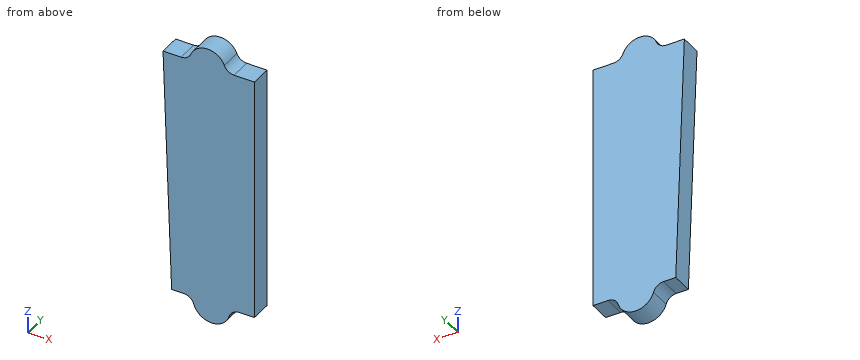
Solid Edge part; units mm, degrees
sketch "Sketch1" plane through (0, 0, 0) normal (0, 0, 1) x (1, 0, 0)
  line L0 (-13, 3) -> (13, 3)
  line L1 (13, 3) -> (13, -3)
  line L2 (13, -3) -> (-13, -3)
  line L3 (-13, -3) -> (-13, 3)
  dimension "D1" = 13
  dimension "D2" = 13
extrude "Protrusion1" add sketch "Sketch1" along normal blind 70
draft "Draft_2" angle 2 neutral plane through (0, 0, 70) normal (0, 0, 1) pull direction (0, 0, -1) face at (-13, -2.06, 57.6333)
sketch "Sketch2" plane through (0, 0, 0) normal (0, -1, 0) x (1, 0, 0)
  line L0 (-5.4345, 70) -> (4.8202, 70)
  arc A0 (-5.4345, 70) -> (4.8202, 70) centre (-0.3072, 69.9621) cw
  line L1 (-4.3885, 0) -> (6.0113, 0)
  arc A1 (-4.3885, 0) -> (6.0113, 0) centre (0.8114, -0.6752) ccw
extrude "ExtrudedProtrusion_2" add sketch "Sketch2" along normal mid plane 6
fillet "Round_1" radius 3 4 edges at (4.8202, 0, 70) (-5.4345, 0, 70) (6.0113, 0, 0) (-4.3885, 0, 0)
properties part number "3"
Here's how the part is built. I have some questions about the finished solid (model axes, mm). Round coordinates to 2 decimals unless told otherwise and drop trailing zeros. Order: outer loops, then holes, each group sorted by start corner. A loop starts at its lowest first (then second) coordinate and runs counter-clockwise, first axis right, second up. Notation, with made-up numbers: (-1, -18.5) -> (11, -18.5) arc R20 cw to (11, 10.5) -> close; hole circle Ø6 at (39, 10.25). An arc over 180 degrees is marked (long way). Use a Markdown table: item, result. Add a question column.
(1) Suppose I cut it at B-B, the plane x = -6.25. Please give me the cut outline in (y, z), and give its area (3 significant figures).
(2) Suppose I cut it at C-C, the plane z = 17.5. Please give me the cut outline in (x, y).
(3) I need wall thicknesses on line 1 along Z through (x, y) = (-10.5, 2.4); line 2 along Z through (x, y) = (-1.5, -0.05); line 3 along X through (y, z) = (-0.25, 45.5). Which ranges of each line are inside material? Lowest first, please.
(4) Suppose I cut it at A-A, the plane y = -1.15. Please give me the cut outline in (x, z), and give its area (3 significant figures).
(5) For pin 1 Ø1.3 at (x, y) = (11.5, 0) entering from -Z; pin 2 Ø1.5 at (x, y) = (-11, -0.5) entering from +Z; pin 3 Ø1.5 at (y, z) = (-2, 19) entering from -X, each with a flat end and sliding along its axis, tell me the tip position at first contact or that it passes through.
Verdict:
| question | item | result |
|---|---|---|
| 1 | outline | (-3, -0.12) -> (3, -0.12) -> (3, 70.46) -> (-3, 70.46) -> close |
| 1 | area | 423 mm2 |
| 2 | outline | (-11.17, -3) -> (13, -3) -> (13, 3) -> (-11.17, 3) -> close |
| 3 | line 1 | 0 to 70 |
| 3 | line 2 | -5.38 to 74.95 |
| 3 | line 3 | -12.14 to 13 |
| 4 | outline | (-13, 70) -> (-10.56, 0) -> (-7.1, 0) arc R3 cw to (-4.22, -2.15) arc R5.24 ccw to (5.84, -2.15) arc R3 cw to (8.72, 0) -> (13, 0) -> (13, 70) -> (7.23, 70) arc R3 cw to (4.45, 71.88) arc R5.13 ccw to (-5.06, 71.88) arc R3 cw to (-7.85, 70) -> close |
| 4 | area | 1,830 mm2 |
| 5 | pin 1 | z = 0 |
| 5 | pin 2 | z = 70 |
| 5 | pin 3 | x = -11.25 |
